Check sheet for the modelled part. Datum: model origin and axes. Units: mm. Face numbers are marked on the shaded views. Round coordinates to 2 decimals unless told otherwise and drop trailing zeros. Order: outer loops, then holes, each group sorted by start corner. A loop starts at its lowest first (then second) coordinate and runs counter-clockwise, first axis right, second up. Notation, with made-up numbers: M -11.5,1.25 L 41.5,1.25 A27 cw 41.5,31.25 Z; hole C 74.5,-35 d5. An arc over 180 degrees is marked long. One line per item, written item: value. Start each with the question number.
(1) Thickness scan on L1, parallel to X at y = 29.8, z = 0; L2, parallel to Z at x = -81.5, y = 36.5; L3, parallel to Y at x = -18, z = -31. Record the ranges inside material, lowest first.
(2) Cross-section at D-D, the plane y = 43.5. Enter the section's corners in (x, z).
(3) Release check for a two-part mould opening along X. For the marked faces 1, 2 and 3 record: released by +X, released by -X, zero draft, split by the parting line, or undercut.
(4) Cross-section at B-B, the plane x = -8.5. Enter the section's corners in (y, z).
(5) Depth check by flat-ended pin: pin 1 Ø3 at (y, z) = (39, -4) entering from +X; pin 2 Ø5.5 at (x, y) = (-86, 62) entering from +Z; pin 3 Ø2.5 at (x, z) = (17.3, 0) entering from -Y. Enter the tip coordinate at first touch or a pass-through.
(6) Cross-section at A-A, the plane z = -15. Enter the section's corners in (x, y), and give its area (3 significant figures).
(7) Cross-section at C-C, the plane y = 61. Enter the section's corners in (x, z).
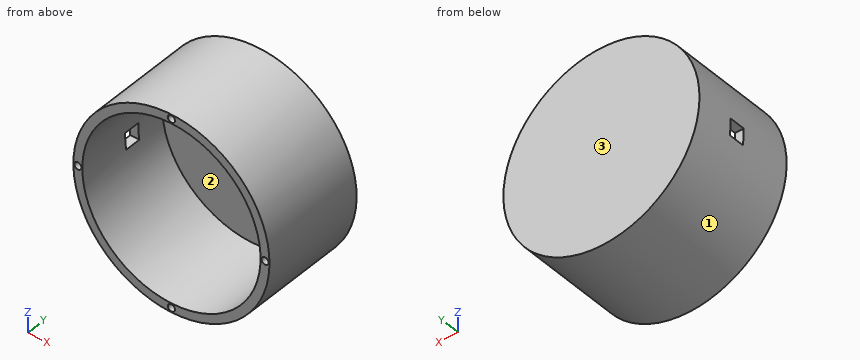
from build123d import *

# Parameters (mm, degrees)
SKETCH2_W          = 55
SKETCH2_H          = 60
SKETCH3_R          = 50
CUT_EXTRUDE1_DEPTH = 55
CUT_EXTRUDE2_DEPTH = 55
SKETCH6_R          = 1.998127765
CUT_EXTRUDE3_DEPTH = 5


with BuildPart() as part:
    # Sketch2 → Revolve1 (revolve)
    with BuildSketch(Plane.XY, mode=Mode.PRIVATE) as revolve1_sk:
        with Locations((-62.704631046, 58.675948718)):
            Rectangle(SKETCH2_W, SKETCH2_H)
    revolve(revolve1_sk.sketch.rotate(Axis((-35.204631046, 28.675948718, 0), (0, 1, 0)), 270), axis=Axis((-35.204631046, 28.675948718, 0), (0, 1, 0)))

    # Sketch3 → Cut-Extrude1 (cut)
    with BuildSketch(Plane.XZ.offset(-28.675948718)):
        with Locations(Location((-35.204631046, 0, 0), (0, 0, 270))):
            Circle(SKETCH3_R)
    extrude(amount=-CUT_EXTRUDE1_DEPTH, mode=Mode.SUBTRACT)

    # Sketch5 → Cut-Extrude2 (cut)
    with BuildSketch(Plane(origin=(-95, 0, 0), x_dir=(0, 0, -1), z_dir=(1, 0, 0))):
        Polygon((3.193764138, 58.175948718), (7.693764138, 58.175948718), (7.693764138, 67.175948718), (-1.306235862, 67.175948718), (-1.306235862, 58.175948718), align=None)
    extrude(amount=CUT_EXTRUDE2_DEPTH, mode=Mode.SUBTRACT)

    # Sketch6 → Cut-Extrude3 (cut)
    with BuildSketch(Plane(origin=(0, 28.675948718, 0), x_dir=(-1, 0, 0), z_dir=(0, -1, 0))):
        with Locations(Location((35.204631046, -52.509597986, 0), (0, 0, 90))):
            Circle(SKETCH6_R)
        with Locations(Location((-17.304966941, 0, 0), (0, 0, 90))):
            Circle(SKETCH6_R)
        with Locations(Location((35.204631046, 52.509597986, 0), (0, 0, 90))):
            Circle(SKETCH6_R)
        with Locations(Location((87.714229032, 0, 0), (0, 0, 90))):
            Circle(SKETCH6_R)
    extrude(amount=-CUT_EXTRUDE3_DEPTH, mode=Mode.SUBTRACT)


solid = part.part
Values found:
1. L1: -90.2 to -89.71, -85.72 to -85.2, 14.8 to 15.31, 19.3 to 19.8
1. L2: -29.69 to -18.89, 18.89 to 29.69
1. L3: 83.68 to 88.68
2. outline: C -35.2,0 d110; hole C -35.2,0 d100
3. face 1: split by the parting line
3. face 2: undercut
3. face 3: zero draft
4. outline: M 28.68,-48.08 L 88.68,-48.08 L 88.68,48.08 L 28.68,48.08 L 28.68,42.27 L 83.68,42.27 L 83.68,-42.27 L 28.68,-42.27 Z
5. pin 1: x = 19.74
5. pin 2: z = 26.77
5. pin 3: y = 33.68
6. outline: M -88.12,28.68 L -82.9,28.68 L -82.9,83.68 L 12.49,83.68 L 12.49,28.68 L 17.71,28.68 L 17.71,88.68 L -88.12,88.68 Z
6. area: 1,100 mm^2
7. outline: M -90.19,1.31 L -85.19,1.31 A50 cw long -84.61,-7.69 L -89.66,-7.69 A55 ccw long Z
